Geometry check sheet. Reference: the model listing, model coordinates, mm. Round coordinates to 2 decimals unless told otherwise and drop trailing zeros. Order: outer loops, then holes, each group sorted by start corner. A loop starts at its lowest first (then second) coordinate and runs counter-clockwise, first axis right, second up. Notation, with made-up numbers: (1.25, 71.25) - (44.25, 71.25) arc R28 ccw to (44.25, 108.25) - close; hole circle Ø8 at (16.25, 44). An arc over 180 degrees is marked (long way). Use a Markdown table: item, result. Add a question column.
(1) Section check A-A on y = 100. Record the boundary of the cut face in (x, z) (3 decimals), then the cut area to 3 significant figures.
(2) Section check B-B on y = 57.5. Record the boundary of the cut face in (x, z), then the cut area to 3 significant figures.
(3) Gauge pin test, flat end, axial feed: P1, Ø6.5, axis at x = -71.42, y = 147.5, coming from the -Z side. Record the tip position at first contact, or that the pin passes through.
(4) Thickness scan on line 1 along X through (y, z) = (-77.5, 10.25). Record the ranges inside material, lowest first. Write a range as [from, to].
(5) Section check C-C on y = 13. Record the boundary of the cut face in (x, z), then the cut area to 3 significant figures.
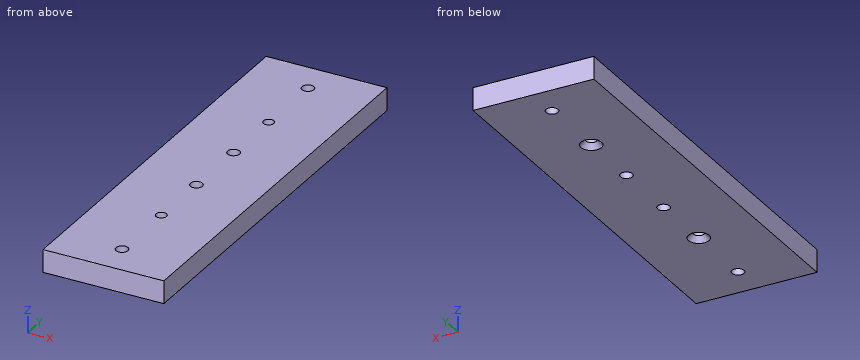
Solid Edge part; units mm, degrees
sketch "Sketch1" plane through (0, 0, 0) normal (0, 0, 1) x (1, 0, 0)
  line L0 (-111.4238, -100) -> (-31.4238, -100)
  line L1 (-31.4238, -100) -> (-31.4238, 170)
  line L2 (-31.4238, 170) -> (-111.4238, 170)
  line L3 (-111.4238, 170) -> (-111.4238, -100)
  dimension "D1" = 31.4238
  dimension "D2" = 31.4238
extrude "Protrusion1" add sketch "Sketch1" along normal blind 15
hole "Agujero_1" at (-71.4238, 100, 0) direction (0, 0, 1) diameter 7 end up to next countersink diameter 13.71 countersink angle 90
hole "Hole1" at (-71.4238, -30, 0) direction (0, 0, 1) diameter 7 end up to next countersink diameter 13.71 countersink angle 90
hole "Agujero_5" at (-71.4238, -77.5, 15) direction (0, 0, -1) diameter 8 end up to next
hole "Hole2" at (-71.4238, 12.5, 15) direction (0, 0, -1) diameter 8 end up to next
hole "Hole3" at (-71.4238, 57.5, 15) direction (0, 0, -1) diameter 8 end up to next
hole "Hole4" at (-71.4238, 147.5, 15) direction (0, 0, -1) diameter 8 end up to next
properties part number "1983-1100-001"
Check sheet entries:
| question | item | result |
|---|---|---|
| 1 | outline | (-111.424, 0) - (-78.279, 0) - (-74.924, 3.355) - (-74.924, 15) - (-111.424, 15) - close; (-67.924, 3.355) - (-64.569, 0) - (-31.424, 0) - (-31.424, 15) - (-67.924, 15) - close |
| 1 | area | 1,080 mm2 |
| 2 | outline | (-111.42, 0) - (-75.42, 0) - (-75.42, 15) - (-111.42, 15) - close; (-67.42, 0) - (-31.42, 0) - (-31.42, 15) - (-67.42, 15) - close |
| 2 | area | 1,080 mm2 |
| 3 | P1 | passes through |
| 4 | line 1 | x = [-111.42, -75.42], [-67.42, -31.42] |
| 5 | outline | (-111.42, 0) - (-75.39, 0) - (-75.39, 15) - (-111.42, 15) - close; (-67.46, 0) - (-31.42, 0) - (-31.42, 15) - (-67.46, 15) - close |
| 5 | area | 1,080 mm2 |
